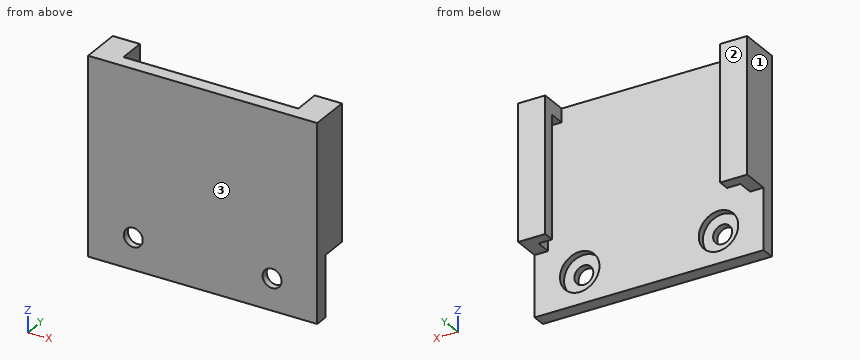
Autodesk Inventor part; units mm, degrees
ref_plane "Work Plane1" through (0, 3.302, 0) normal (0, 1, 0) x (1, 0, 0)
ref_plane "Work Plane2" through (0, 4.572, 0) normal (0, 1, 0) x (1, 0, 0)
ref_plane "Work Plane3" through (0, 1.524, 0) normal (0, 1, 0) x (1, 0, 0)
sketch "Sketch1" plane through (0, 0, 0) normal (0, 1, 0) x (-1, 0, 0)
  line L0 (0, 0) -> (-25.781, 0)
  line L1 (-25.781, 0) -> (-25.781, -22.098)
  line L2 (-25.781, -22.098) -> (0, -22.098)
  line L3 (0, -22.098) -> (0, 0)
  line L4 (-1.524, -20.574) -> (-24.257, -20.574)
  line L5 (-24.257, -20.574) -> (-24.257, -1.524)
  line L6 (-24.257, -1.524) -> (-1.524, -1.524)
  line L7 (-1.524, -1.524) -> (-1.524, -20.574)
  line L8 (-3.048, 0) -> (-3.048, -1.524)
  line L9 (-22.733, 0) -> (-22.733, -1.524)
  line L10 (-3.048, -20.574) -> (-3.048, -22.098)
  line L11 (-3.048, -1.524) -> (-3.048, -20.574)
  line L12 (-22.733, -1.524) -> (-22.733, -20.574)
  line L13 (-22.733, -20.574) -> (-22.733, -22.098)
  line L14 (0, -15.24) -> (-1.524, -15.24)
  line L15 (-24.257, -15.24) -> (-25.781, -15.24)
  line L16 (-1.524, -15.24) -> (-3.048, -15.24)
  line L17 (-24.257, -15.24) -> (-22.733, -15.24)
  circle A0 centre (-5.08, -18.542) radius 1.0668
  circle A1 centre (-20.701, -2.032) radius 1.0668
  circle A2 centre (-20.701, -18.542) radius 1.0668
  circle A3 centre (-5.08, -2.032) radius 1.0668
  dimension "d2" = 1.524
  dimension "d3" = 19.05
  dimension "d4" = 22.733
  dimension "d5" = 1.524
  dimension "d6" = 1.524
  dimension "d10" = 6.858
  dimension "d11" = 6.858
  dimension "d19" = 2.1336
  dimension "d22" = 2.032
  dimension "d23" = 2.032
  dimension "d24" = 2.032
  dimension "d25" = 16.51
  dimension "d26" = 16.51
extrude "Extrusion2" add sketch "Sketch1" along normal blind 3.302 contours L3 L14 L7 L6 L8 L0 | L9 L6 L5 L15 L1 L0
ref_plane "Work Plane1" through (0, 3.302, 0) normal (0, 1, 0) x (1, 0, 0)
ref_plane "Work Plane2" through (0, 4.572, 0) normal (0, 1, 0) x (1, 0, 0)
extrude "Extrusion3" add sketch "Sketch1" along normal up to surface (1.27 mm away) from surface at 3.302 contours L3 L14 L7 L6 L8 L0 | L9 L6 L5 L15 L1 L0 | L6 L7 L16 L11 | L12 L17 L5 L6
ref_plane "Work Plane3" through (0, 1.524, 0) normal (0, 1, 0) x (1, 0, 0)
sketch "Sketch2" plane through (0, 1.524, 0) normal (0, 1, 0) x (1, 0, 0)
  circle A0 centre (5.08, 18.542) radius 1.0668
  circle A1 centre (20.701, 18.542) radius 1.0668
  circle A2 centre (20.701, 2.032) radius 1.0668
  circle A3 centre (5.08, 2.032) radius 1.0668
  circle A4 centre (20.701, 2.032) radius 1.0668
  circle A5 centre (20.701, 18.542) radius 1.0668
  point P0 (0, 0)
extrude "Extrusion7" add sketch "Sketch1" along normal blind 1.524 contours L8 L6 A3 A1 L9 L0 | L3 L2 L10 L4 L7 L14 | L11 L4 L12 L6 A1 A3 | L6 L7 L16 L11 | L7 L4 L11 L16 | L12 L17 L5 L6 | A3 L6 | L6 A3 | L2 L13 L4 L10 | L15 L5 L4 L13 L2 L1 | A1 L6 | L6 A1 | L12 L4 L5 L17
hole "Hole2" at (20.701, 1.524, -18.542) at (5.08, 1.524, -18.542) direction (0, -1, 0) diameter 0.4763 end through all counterbore diameter 4.445 counterbore depth 0.762
properties part number "ShockSensorMount" material "Glass"
Geometry: final body of the model. Coordinates: model frame, mm. Face numbers are marked on the shaded views. Give positions to 0.01 mm unless a question says otherwise; leave off trailing zeros. Order: outer loops, then holes, each group sorted by start corner. A loop starts at its lowest first (then second) coordinate and runs counter-clockwise, first axis right, second up. Notation, with made-up numbers: (36, 52) -> (47, 52) arc R13 ccw to (47, 65) -> close; hole circle Ø7 at (81, 22.5). An arc over 180 degrees is marked (long way). Put each result on its own line as item: value.
Q1. Pin query (flat end, axial travel): pin 1 (3.5 mm diameter, centred on x = 22, z = -18, fed in from +Y); pin 2 (0.9 mm diameter, centred on x = 2, y = 3, fed in from -Z); pin 3 (0.5 mm diameter, centred on x = 23, y = 2.5, fed in from -Z). Return the tip coordinate at first contact, or that it passes through.
Here are the results:
pin 1: stops at y = 1.52
pin 2: stops at z = -15.24
pin 3: stops at z = -1.52
Q2. Section A-A, the plane x = 5.08. Return loops of the section in (y, z), then the cut area to 3 significant figures.
Here are the results:
outline: (0, -22.1) -> (1.52, -22.1) -> (1.52, -20.76) -> (0.76, -20.76) -> (0.76, -19.61) -> (0, -19.61) -> close; (0, -17.48) -> (0.76, -17.48) -> (0.76, -16.32) -> (1.52, -16.32) -> (1.52, 0) -> (0, 0) -> close
area: 28.7 mm^2
Q3. Section C-C, the plane x = 12.75. Return loops of the section in (y, z), then the cut area to 3 significant figures.
Here are the results:
outline: (0, -22.1) -> (1.52, -22.1) -> (1.52, 0) -> (0, 0) -> close
area: 33.7 mm^2
Q4. Draft query along Y for the marked faces 1, 2 and 3. Return one class per face: released by +Y, released by -Y, zero draft, split by the parting line, or undercut.
Here are the results:
face 1: zero draft
face 2: released by +Y
face 3: released by -Y
Q5. Section B-B, the plane z = -3.5. Return loops of the section in (x, y).
Here are the results:
outline: (0, 0) -> (25.78, 0) -> (25.78, 4.57) -> (22.73, 4.57) -> (22.73, 3.3) -> (24.26, 3.3) -> (24.26, 1.52) -> (1.52, 1.52) -> (1.52, 3.3) -> (3.05, 3.3) -> (3.05, 4.57) -> (0, 4.57) -> close
Q6. Material intervals for L1, parallel to X at y = 4.2, z = -12.5; L2, parallel to Z at x = 5.08, y = 0.45; L3, parallel to X at y = 2.4, z = -10, sorted ascending.
Here are the results:
L1: x = 0 to 3.05, 22.73 to 25.78
L2: z = -22.1 to -19.61, -17.48 to 0
L3: x = 0 to 1.52, 24.26 to 25.78
